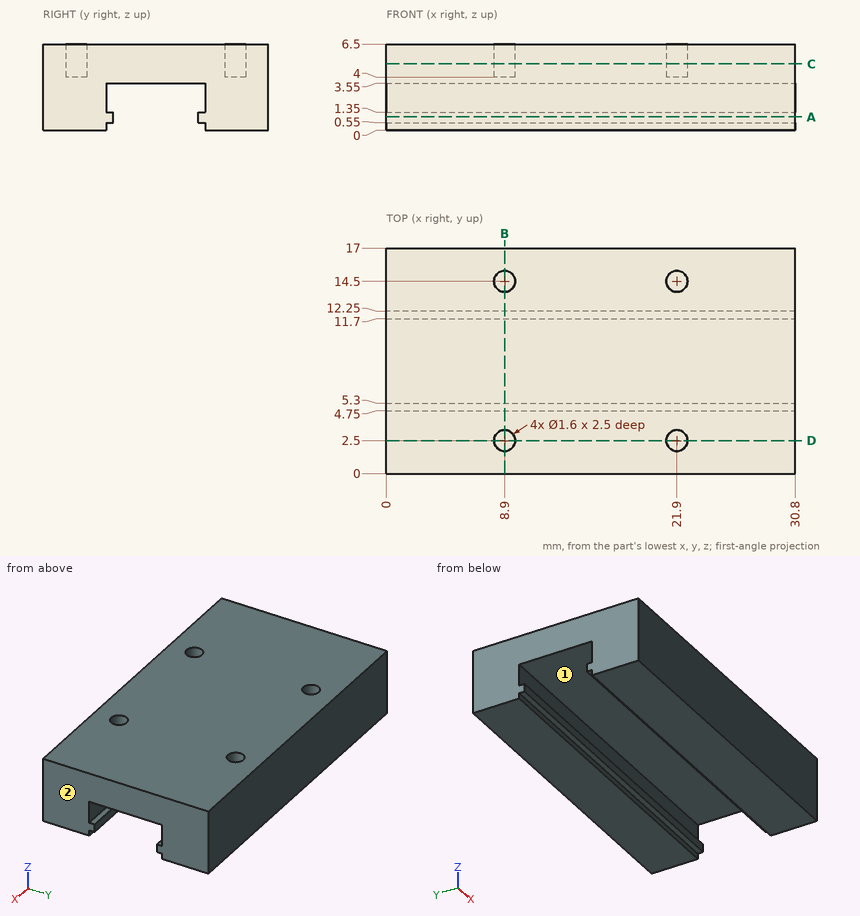
The drawing under review shows one solid part. Ordinate dimensions are in mm from its lowest x, y, z. A direction names the side the tool comes from. Give positions to 0.01 mm unless a question says otherwise; leave off trailing zeros. Order: outer loops, then holes, each group sorted by start corner. A loop starts at its lowest first (then second) coordinate and runs counter-clockwise, first axis right, second up. Notation, with made-up numbers: M 81,78 L 108,78 A20 ccw 108,112 Z; hole C 59.25,56 d6. An arc over 180 degrees is marked long. One line per question, with ' | ' between items. Start each with the question number.
Q1. For pin 1 Ø5 at (x, y) = (23.5, 9.5) entering from -Z; pin 2 Ø1.4 at (x, y) = (8.9, 2.5) entering from +Z, all flat-tipped, find the tip position at first contact; note any pin that passes through.
Q2. Machinability: for the marked faces 1 and 2, which of the approach directions +Z, -Z, +X, -X, +Y, -Y give a long, thin tool a straight path to every point of the face, cutting with its end or side? Answer none if there is none.
Q3. We need section D-D (y = 2.5). Write out the cut boundary in (x, z).
Q4. For L1, parallel to X at y = 14.5, z = 5.25; L2, parallel to Y at x = 21.9, z = 5.65; L3, parallel to Y at x = 24, z = 3.5, list the stretches that pass through material, from the lowest coordinate up. Write a range as [from, to].
Q5. We need section B-B (x = 8.9). Write out the cut boundary in (y, z).
Q6. We need section A-A (z = 1). Write out the cut boundary in (x, y), plus the area to 3 significant figures.
Q7. We need section C-C (z = 5). Write out the cut boundary in (x, y).
Returned:
1) pin 1: z = 0.55 | pin 2: z = 4
2) face 1: +X, -X | face 2: +Z, -Z, +X, +Y, -Y
3) outline: M 0,0 L 30.8,0 L 30.8,6.5 L 22.7,6.5 L 22.7,4 L 21.1,4 L 21.1,6.5 L 9.7,6.5 L 9.7,4 L 8.1,4 L 8.1,6.5 L 0,6.5 Z
4) L1: [0, 8.1], [9.7, 21.1], [22.7, 30.8] | L2: [0, 1.7], [3.3, 13.7], [15.3, 17] | L3: [0, 4.75], [12.25, 17]
5) outline: M 0,0 L 4.75,0 L 4.75,0.55 L 5.3,0.55 L 5.3,1.35 L 4.75,1.35 L 4.75,3.55 L 12.25,3.55 L 12.25,1.35 L 11.7,1.35 L 11.7,0.55 L 12.25,0.55 L 12.25,0 L 17,0 L 17,6.5 L 15.3,6.5 L 15.3,4 L 13.7,4 L 13.7,6.5 L 3.3,6.5 L 3.3,4 L 1.7,4 L 1.7,6.5 L 0,6.5 Z
6) outline: M 0,0 L 30.8,0 L 30.8,5.3 L 0,5.3 Z; M 0,11.7 L 30.8,11.7 L 30.8,17 L 0,17 Z | area: 326 mm2
7) outline: M 0,0 L 30.8,0 L 30.8,17 L 0,17 Z; hole C 8.9,2.5 d1.6; hole C 8.9,14.5 d1.6; hole C 21.9,2.5 d1.6; hole C 21.9,14.5 d1.6
